Geometry check sheet. Reference: the model listing, model coordinates, mm. Face numbers are marked on the shaded views. A direction names the side the tool comes from. Coordinates: 2 decimals unless noted, no trailing zeros. Loops run counter-clockwise (first coordinate to the right, second up) from the corner with the lowest first, then second, coordinate; pieces in that order, holes last. Notation, with made-up numbers: (-14, 35.25) - (16, 35.25) arc R16 cw to (16, 40.25) - close; hole circle Ø6 at (32.25, -4.5). An arc over 180 degrees is marked (long way). One line per item, written item: value.
Autodesk Inventor part; units mm, degrees
ref_plane "Work Plane1" through (0, 1, 0) normal (0, 1, 0) x (-1, 0, 0)
ref_plane "YZ Plane" through (0, 0, 0) normal (1, 0, 0) x (0, 1, 0)
ref_plane "XY Plane" through (0, 0, 0) normal (0, 0, 1) x (1, 0, 0)
sketch "Sketch1" plane through (0, 0, 0) normal (0, 1, 0) x (-1, 0, 0)
  circle A0 centre (0, 0) radius 12.5
  dimension "d0" = 25
extrude "Extrusion1" add sketch "Sketch1" along normal blind 4.5
ref_plane "Work Plane1" through (0, 1, 0) normal (0, 1, 0) x (-1, 0, 0)
sketch "Sketch2" plane through (0, 1, 0) normal (0, 1, 0) x (-1, 0, 0)
  line L0 (15, -1) -> (-15, -1)
  arc A0 (21, -27) -> (15, -1) centre (-24.8954, -23.8989) ccw
  line L1 (21, -27) -> (-21, -27)
  arc A1 (-15, -1) -> (-21, -27) centre (24.8954, -23.8989) ccw
  line L2 (-19.6045, -25.5298) -> (19.6045, -25.5298)
  arc A2 (19.6045, -25.5298) -> (14.1394, -2.4702) centre (-24.8954, -23.8989) ccw
  line L3 (14.1394, -2.4702) -> (-14.1394, -2.4702)
  arc A3 (-14.1394, -2.4702) -> (-19.6045, -25.5298) centre (24.8954, -23.8989) ccw
  line L4 (31.9342, 0) -> (-23.3502, 0) construction
  line L5 (15, 1) -> (-15, 1)
  arc A4 (15, 1) -> (21, 27) centre (-24.8954, 23.8989) ccw
  line L6 (21, 27) -> (-21, 27)
  arc A5 (-21, 27) -> (-15, 1) centre (24.8954, 23.8989) ccw
  line L7 (-19.6045, 25.5298) -> (19.6045, 25.5298)
  arc A6 (14.1394, 2.4702) -> (19.6045, 25.5298) centre (-24.8954, 23.8989) ccw
  line L8 (14.1394, 2.4702) -> (-14.1394, 2.4702)
  arc A7 (-19.6045, 25.5298) -> (-14.1394, 2.4702) centre (24.8954, 23.8989) ccw
  point P0 (0, 0)
  point P1 (0, -1)
  point P2 (0, -27)
  point P3 (0, 1)
  point P4 (0, 27)
  dimension "d4" = 1
  dimension "d5" = 30
  dimension "d6" = 26
  dimension "d7" = 42
  dimension "d8" = 46
  dimension "d9" = 46
extrude "Extrusion2" add sketch "Sketch2" along normal blind 2.65
fillet "Fillet1" radius 2 1 edges at (12.5, 4.5, 0)
sketch "Sketch3" plane through (0, 0, 0) normal (0, -1, 0) x (1, 0, 0)
  line L0 (-7.886, 0) -> (-6.3799, 4.6353)
  line L1 (-6.3799, 4.6353) -> (-2.4369, 7.5)
  line L2 (-2.4369, 7.5) -> (2.4369, 7.5)
  line L3 (2.4369, 7.5) -> (6.3799, 4.6353)
  line L4 (6.3799, 4.6353) -> (7.886, 0)
  line L5 (7.886, 0) -> (6.3799, -4.6353)
  line L6 (6.3799, -4.6353) -> (2.4369, -7.5)
  line L7 (2.4369, -7.5) -> (-2.4369, -7.5)
  line L8 (-2.4369, -7.5) -> (-6.3799, -4.6353)
  line L9 (-6.3799, -4.6353) -> (-7.886, 0)
  point P0 (0, 0)
  point P1 (0, 0)
  point P2 (0, -7.5)
  dimension "d13" = 15
extrude "Extrusion3" add sketch "Sketch3" along normal blind 3
properties part number "brace_tabs"
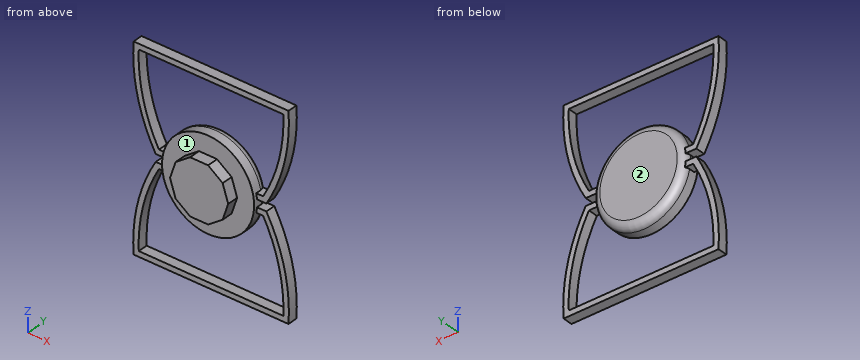
(1) Cross-section at C-C on z = 16. Record the cut outline in (x, y).
Reply:
outline: (-20.42, 1) - (-18.93, 1) - (-18.93, 3.65) - (-20.42, 3.65) - close; (18.93, 1) - (20.42, 1) - (20.42, 3.65) - (18.93, 3.65) - close
(2) Go/stop test with flat-tipped pins: pin 1 Ø8 at (x, z) = (10.5, 12) entering from +Y; pin 2 Ø1.5 at (x, y) = (1, -1) entering from +Z; pin 3 Ø5 at (x, z) = (13.5, -3) entering from +Y. Record where each tip stops, or that it passes through.
Reply:
pin 1: y = 3.88
pin 2: z = 7.5
pin 3: y = 4.32
(3) Cross-section at A-A on x = 0. Record the cut outline in (y, z).
Reply:
outline: (-3, -7.5) - (0, -7.5) - (0, -12.5) - (2.5, -12.5) arc R2 ccw to (4.5, -10.5) - (4.5, 10.5) arc R2 ccw to (2.5, 12.5) - (0, 12.5) - (0, 7.5) - (-3, 7.5) - close; (1, -27) - (3.65, -27) - (3.65, -25.53) - (1, -25.53) - close; (1, 25.53) - (3.65, 25.53) - (3.65, 27) - (1, 27) - close
(4) Material ranges on probe 1 along Z at (x, y) = (-10, 2.25); probe 2 along Z at (x, y) = (-5, 2.75); probe 3 along X at (y, z) = (1.25, 10), recorded low to high. Write a range as from..to.
Reply:
probe 1: -27..-25.53, -7.5..7.5, 25.53..27
probe 2: -27..-25.53, -11.44..11.44, 25.53..27
probe 3: -18.95..-17.41, -7.5..7.5, 17.41..18.95
(5) Cross-section at D-D on z = -6.5. State how many separate pieces and enclosed holes the cut face has, and give its area (3 significant figures).
Reply:
separate pieces: 3
enclosed holes: 0
area: 125 mm2
(6) Cross-section at B-B on y = -1.75. Record the cut outline in (x, z).
Reply:
outline: (-7.89, 0) - (-6.38, -4.64) - (-2.44, -7.5) - (2.44, -7.5) - (6.38, -4.64) - (7.89, 0) - (6.38, 4.64) - (2.44, 7.5) - (-2.44, 7.5) - (-6.38, 4.64) - close
(7) Access from +Z, -Z, +X, -X, +Y, -Y to the whole of each face (thin tool, end or side, straight path). Record for the marked faces 1 and 2.
Reply:
face 1: -Y
face 2: +Z, -Z, +X, -X, +Y
